Part model, mm, in its own coordinate system. Face numbers are marked on the shaded views. A direction names the side the tool comes from. Give positions to 0.01 mm unless a question says otherwise; leave off trailing zeros. Order: outer loops, then holes, each group sorted by start corner. A loop starts at its lowest first (then second) coordinate and runs counter-clockwise, first axis right, second up. Notation, with made-up numbers: M 65,73.25 L 123,73.25 A21 cw 123,106.25 Z; hole C 78,29 d7. An arc over 180 degrees is marked long. Return JSON: item names as keys, results as strings.
from build123d import *

# Parameters (mm, degrees)
SCHIZZO1_R                    = 3.005
ESTRUSIONE_ESTRUSIONE1_DEPTH  = 6.5
SCHIZZO2_R                    = 0.98
ESTRUSIONE_ESTRUSIONE2_DEPTH  = 2.5
SCHIZZO3_R                    = 0.85
ESTRUSIONE_ESTRUSIONE3_DEPTH  = 1
SCHIZZO4_R                    = 0.98
ESTRUSIONE_ESTRUSIONE4_DEPTH  = 2.2
FORO_FILETTATO_M3X0_5_1_D     = 2.5
FORO_FILETTATO_M3X0_5_1_DEPTH = 5
FORO_FILETTATO_M3X0_5_1_TIP   = 0.751075774
TAGLIO_ESTRUSIONE1_DEPTH      = 13.918980223
TAGLIO_ESTRUSIONE1_DEPTH_BACK = 13.918980223
SCHIZZO7_R                    = 0.99


with BuildPart() as part:
    # Schizzo1 → Estrusione-Estrusione1 (new body)
    with BuildSketch(Plane(origin=(0, 0, 0), x_dir=(0, 0, -1), z_dir=(1, 0, 0))):
        with Locations(Location((0, 0, 0), (0, 0, 180))):
            Circle(SCHIZZO1_R)
    extrude(amount=ESTRUSIONE_ESTRUSIONE1_DEPTH)

    # Schizzo2 → Estrusione-Estrusione2 (add)
    with BuildSketch(Plane(origin=(6.5, 0, 0), x_dir=(0, 0, -1), z_dir=(1, 0, 0))):
        Circle(SCHIZZO2_R)
    extrude(amount=ESTRUSIONE_ESTRUSIONE2_DEPTH)

    # Schizzo3 → Estrusione-Estrusione3 (add)
    with BuildSketch(Plane(origin=(9, 0, 0), x_dir=(0, 0, -1), z_dir=(1, 0, 0))):
        Circle(SCHIZZO3_R)
    extrude(amount=ESTRUSIONE_ESTRUSIONE3_DEPTH)

    # Schizzo4 → Estrusione-Estrusione4 (add)
    with BuildSketch(Plane(origin=(10, 0, 0), x_dir=(0, 0, -1), z_dir=(1, 0, 0))):
        Circle(SCHIZZO4_R)
    extrude(amount=ESTRUSIONE_ESTRUSIONE4_DEPTH)

    # Foro filettato M3x0.5-1
    with Locations(Plane.ZY):
        with Locations((0, 0)):
            Hole(FORO_FILETTATO_M3X0_5_1_D / 2, depth=FORO_FILETTATO_M3X0_5_1_DEPTH)
            with Locations((0, 0, -(FORO_FILETTATO_M3X0_5_1_DEPTH + FORO_FILETTATO_M3X0_5_1_TIP / 2))):  # 118° drill point
                Cone(0, FORO_FILETTATO_M3X0_5_1_D / 2, FORO_FILETTATO_M3X0_5_1_TIP, mode=Mode.SUBTRACT)

    # Schizzo7 → Taglio-Estrusione1 (cut, two sides: drawn at the far end of the back side and taken through both)
    with BuildSketch(Plane.XY.offset(-TAGLIO_ESTRUSIONE1_DEPTH_BACK)):
        with Locations((2.99, 0)):
            Circle(SCHIZZO7_R)
    extrude(amount=TAGLIO_ESTRUSIONE1_DEPTH + TAGLIO_ESTRUSIONE1_DEPTH_BACK, mode=Mode.SUBTRACT)


solid = part.part
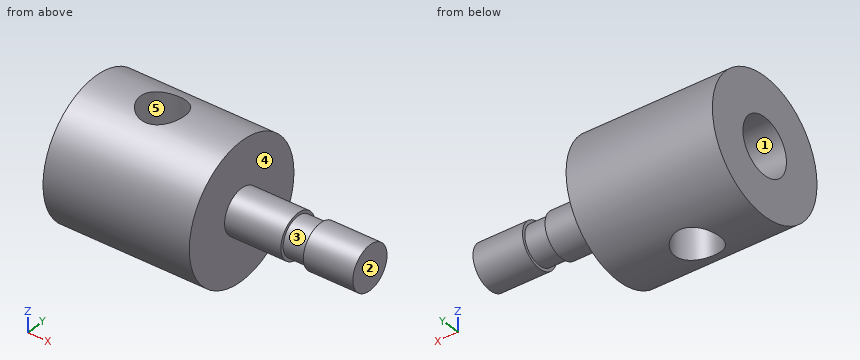
Q1. Pin check, flat tip, straight feed: pin 1 (2 mm diameter, centred on y = 0, z = -0.5, fed in from -X). Stop position of the tip, or through.
Established:
{"pin 1": "stops at x = 0"}
Q2. Band-saw the part on B-B (y = 0.5). Give the number of separate pieces and of enclosed holes in the cut face, then the cut area to 3 significant figures.
Established:
{"separate pieces": "3", "enclosed holes": "0", "area": "29.5 mm²"}
Q3. Probe line 1 along Y through (x, z) = (2.1, 0) (3 decimals); line 2 along X through (y, z) = (0, -2); line 3 along X through (y, z) = (1.75, -1.5). List the from-to ranges inside material, lowest first.
Established:
{"line 1": "y = -3.005 to -1.25, 1.25 to 3.005", "line 2": "x = 0 to 2, 3.98 to 6.5", "line 3": "x = 0 to 6.5"}
Q4. Band-saw the part on C-C (x = 1.25). Give the cut face in (y, z) (3 decimals), then the cut area to 3 significant figures.
Established:
{"outline": "C 0,0 d6.01; hole C 0,0 d2.5", "area": "23.5 mm²"}
Q5. 3-axis set-ups, long thin cutter, end or side, ignore diameter. For the marked faces 4 and 5: which of +Z, -Z, +X, -X, +Y, -Y reach the whole face in a straight line?
Established:
{"face 4": "+X", "face 5": "+Z, -Z"}
Q6. Band-saw the part on D-D (y = -1.75). Give the cut face in (x, z), then the cut area to 3 significant figures.
Established:
{"outline": "M 0,-2.44 L 6.5,-2.44 L 6.5,2.44 L 0,2.44 Z", "area": "31.8 mm²"}
Q7. Band-saw the part on A-A (x = 2.99). Give the cut face in (y, z) (3 decimals), then the cut area to 3 significant figures.
Established:
{"outline": "M -0.99,-2.837 L -0.99,-0.763 A1.25 cw -0.99,0.763 L -0.99,2.837 A3.005 ccw Z; M 0.99,-2.837 A3.005 ccw 0.99,2.837 L 0.99,0.763 A1.25 cw 0.99,-0.763 Z", "area": "16.1 mm²"}
Q8. Two-plate mould, pull along Z, no slides. Class the marked faces 1, 2 and 3: +Z half, -Z half, draft (parallel to the pull), parting line (faces both ways), or undercut.
Established:
{"face 1": "undercut", "face 2": "draft", "face 3": "parting line"}
